from build123d import *

# Parameters (mm, degrees)
F1_DEPTH = 8
F3_DEPTH = 1
F5_DEPTH = 25


with BuildPart() as f1:
    # F0 (on Top) → F1 (new body)
    with BuildSketch(Plane.XY):
        with BuildLine():
            Line((77.8597715207, -29.7489808303), (77.8597715207, 29.7489808303))
            Line((77.8597715207, 29.7489808303), (-77.8597715207, 29.7489808303))
            Line((-77.8597715207, 29.7489808303), (-77.8597715207, -29.7489808303))
            Line((-77.8597715207, -29.7489808303), (-67.8597715207, -29.7489808303))
            Line((-67.8597715207, -29.7489808303), (-67.8597715207, -16.2489808303))
            ThreePointArc((-67.8597715207, -16.2489808303), (-68.9204316925, -13.6883206586), (-66.3597715207, -14.7489808303))
            Line((-66.3597715207, -14.7489808303), (-41.3597715207, -14.7489808303))
            ThreePointArc((-41.3597715207, -14.7489808303), (-38.7991113489, -13.6883206586), (-39.8597715207, -16.2489808303))
            Line((-39.8597715207, -16.2489808303), (-39.8597715207, -29.7489808303))
            Line((-39.8597715207, -29.7489808303), (77.8597715207, -29.7489808303))
        make_face()
        with BuildLine():
            Line((-67.8597715207, -29.7489808303), (-39.8597715207, -29.7489808303))
            Line((-39.8597715207, -29.7489808303), (-39.8597715207, -16.2489808303))
            ThreePointArc((-39.8597715207, -16.2489808303), (-38.7991113489, -13.6883206586), (-41.3597715207, -14.7489808303))
            Line((-41.3597715207, -14.7489808303), (-66.3597715207, -14.7489808303))
            ThreePointArc((-66.3597715207, -14.7489808303), (-68.9204316925, -13.6883206586), (-67.8597715207, -16.2489808303))
            Line((-67.8597715207, -16.2489808303), (-67.8597715207, -29.7489808303))
        make_face()
    extrude(amount=F1_DEPTH)

    # F2 (on face) → F3 (join)
    with BuildSketch(Plane.XY.offset(8)):
        with BuildLine():
            Line((-67.8597715207, -16.2489808303), (-67.8597715207, -29.7489808303))
            Line((-67.8597715207, -29.7489808303), (-39.8597715207, -29.7489808303))
            Line((-39.8597715207, -29.7489808303), (-39.8597715207, -16.2489808303))
            ThreePointArc((-39.8597715207, -16.2489808303), (-38.7991113489, -13.6883206586), (-41.3597715207, -14.7489808303))
            Line((-41.3597715207, -14.7489808303), (-66.3597715207, -14.7489808303))
            ThreePointArc((-66.3597715207, -14.7489808303), (-68.9204316925, -13.6883206586), (-67.8597715207, -16.2489808303))
        make_face()
    extrude(amount=F3_DEPTH)

    # F4 (on face) → F5 (cut)
    with BuildSketch(Plane.XY.offset(9)):
        with BuildLine():
            ThreePointArc((-62.6597715207, -18.936415039), (-62.9597715207, -17.7489808303), (-62.6597715207, -16.5615466216))
            ThreePointArc((-62.6597715207, -16.5615466216), (-67.3597715207, -17.7489808303), (-62.6597715207, -18.936415039))
        make_face()
        with BuildLine():
            ThreePointArc((-62.6597715207, -16.5615466216), (-62.435931592, -17.1366083946), (-62.3597715207, -17.7489808303))
            ThreePointArc((-62.3597715207, -17.7489808303), (-62.435931592, -18.361353266), (-62.6597715207, -18.936415039))
            ThreePointArc((-62.6597715207, -18.936415039), (-60.4597715207, -20.2489808303), (-58.2597715207, -18.936415039))
            ThreePointArc((-58.2597715207, -18.936415039), (-58.5597715207, -17.7489808303), (-58.2597715207, -16.5615466216))
            ThreePointArc((-58.2597715207, -16.5615466216), (-60.4597715207, -15.2489808303), (-62.6597715207, -16.5615466216))
        make_face()
        with BuildLine():
            ThreePointArc((-53.8597715207, -16.5615466216), (-56.0597715207, -15.2489808303), (-58.2597715207, -16.5615466216))
            ThreePointArc((-58.2597715207, -16.5615466216), (-58.035931592, -17.1366083946), (-57.9597715207, -17.7489808303))
            ThreePointArc((-57.9597715207, -17.7489808303), (-58.035931592, -18.361353266), (-58.2597715207, -18.936415039))
            ThreePointArc((-58.2597715207, -18.936415039), (-56.0597715207, -20.2489808303), (-53.8597715207, -18.936415039))
            ThreePointArc((-53.8597715207, -18.936415039), (-54.1597715207, -17.7489808303), (-53.8597715207, -16.5615466216))
        make_face()
        with BuildLine():
            ThreePointArc((-49.4597715207, -16.5615466216), (-51.6597715207, -15.2489808303), (-53.8597715207, -16.5615466216))
            ThreePointArc((-53.8597715207, -16.5615466216), (-53.635931592, -17.1366083946), (-53.5597715207, -17.7489808303))
            ThreePointArc((-53.5597715207, -17.7489808303), (-53.635931592, -18.361353266), (-53.8597715207, -18.936415039))
            ThreePointArc((-53.8597715207, -18.936415039), (-51.6597715207, -20.2489808303), (-49.4597715207, -18.936415039))
            ThreePointArc((-49.4597715207, -18.936415039), (-49.7597715207, -17.7489808303), (-49.4597715207, -16.5615466216))
        make_face()
        with BuildLine():
            ThreePointArc((-45.0597715207, -16.5615466216), (-47.2597715207, -15.2489808303), (-49.4597715207, -16.5615466216))
            ThreePointArc((-49.4597715207, -16.5615466216), (-49.235931592, -17.1366083946), (-49.1597715207, -17.7489808303))
            ThreePointArc((-49.1597715207, -17.7489808303), (-49.235931592, -18.361353266), (-49.4597715207, -18.936415039))
            ThreePointArc((-49.4597715207, -18.936415039), (-47.2597715207, -20.2489808303), (-45.0597715207, -18.936415039))
            ThreePointArc((-45.0597715207, -18.936415039), (-45.3597715207, -17.7489808303), (-45.0597715207, -16.5615466216))
        make_face()
        with BuildLine():
            ThreePointArc((-40.3597715207, -17.7489808303), (-42.247399085, -15.3251409016), (-45.0597715207, -16.5615466216))
            ThreePointArc((-45.0597715207, -16.5615466216), (-44.835931592, -17.1366083946), (-44.7597715207, -17.7489808303))
            ThreePointArc((-44.7597715207, -17.7489808303), (-44.835931592, -18.361353266), (-45.0597715207, -18.936415039))
            ThreePointArc((-45.0597715207, -18.936415039), (-42.247399085, -20.1728207591), (-40.3597715207, -17.7489808303))
        make_face()
        with BuildLine():
            ThreePointArc((-57.9597715207, -17.7489808303), (-58.035931592, -17.1366083946), (-58.2597715207, -16.5615466216))
            ThreePointArc((-58.2597715207, -16.5615466216), (-58.5597715207, -17.7489808303), (-58.2597715207, -18.936415039))
            ThreePointArc((-58.2597715207, -18.936415039), (-58.035931592, -18.361353266), (-57.9597715207, -17.7489808303))
        make_face()
        with BuildLine():
            ThreePointArc((-62.6597715207, -18.936415039), (-62.435931592, -18.361353266), (-62.3597715207, -17.7489808303))
            ThreePointArc((-62.3597715207, -17.7489808303), (-62.435931592, -17.1366083946), (-62.6597715207, -16.5615466216))
            ThreePointArc((-62.6597715207, -16.5615466216), (-62.9597715207, -17.7489808303), (-62.6597715207, -18.936415039))
        make_face()
        with BuildLine():
            ThreePointArc((-53.5597715207, -17.7489808303), (-53.635931592, -17.1366083946), (-53.8597715207, -16.5615466216))
            Line((-53.8597715207, -16.5615466216), (-53.8597715207, -18.936415039))
            ThreePointArc((-53.8597715207, -18.936415039), (-53.635931592, -18.361353266), (-53.5597715207, -17.7489808303))
        make_face()
        with BuildLine():
            ThreePointArc((-49.1597715207, -17.7489808303), (-49.235931592, -17.1366083946), (-49.4597715207, -16.5615466216))
            ThreePointArc((-49.4597715207, -16.5615466216), (-49.7597715207, -17.7489808303), (-49.4597715207, -18.936415039))
            ThreePointArc((-49.4597715207, -18.936415039), (-49.235931592, -18.361353266), (-49.1597715207, -17.7489808303))
        make_face()
        with BuildLine():
            ThreePointArc((-44.7597715207, -17.7489808303), (-44.835931592, -17.1366083946), (-45.0597715207, -16.5615466216))
            ThreePointArc((-45.0597715207, -16.5615466216), (-45.3597715207, -17.7489808303), (-45.0597715207, -18.936415039))
            ThreePointArc((-45.0597715207, -18.936415039), (-44.835931592, -18.361353266), (-44.7597715207, -17.7489808303))
        make_face()
        with BuildLine():
            Line((-53.8597715207, -18.936415039), (-53.8597715207, -16.5615466216))
            ThreePointArc((-53.8597715207, -16.5615466216), (-54.1597715207, -17.7489808303), (-53.8597715207, -18.936415039))
        make_face()
        with BuildLine():
            ThreePointArc((-67.8597715207, -16.2489808303), (-66.7991113489, -15.8096410021), (-66.3597715207, -14.7489808303))
            ThreePointArc((-66.3597715207, -14.7489808303), (-68.9204316925, -13.6883206586), (-67.8597715207, -16.2489808303))
        make_face()
        with BuildLine():
            ThreePointArc((-38.3597715207, -14.7489808303), (-39.8597715207, -13.2489808303), (-41.3597715207, -14.7489808303))
            ThreePointArc((-41.3597715207, -14.7489808303), (-40.9204316925, -15.8096410021), (-39.8597715207, -16.2489808303))
            ThreePointArc((-39.8597715207, -16.2489808303), (-38.7991113489, -15.8096410021), (-38.3597715207, -14.7489808303))
        make_face()
    extrude(amount=-F5_DEPTH, mode=Mode.SUBTRACT)


solid = f1.part
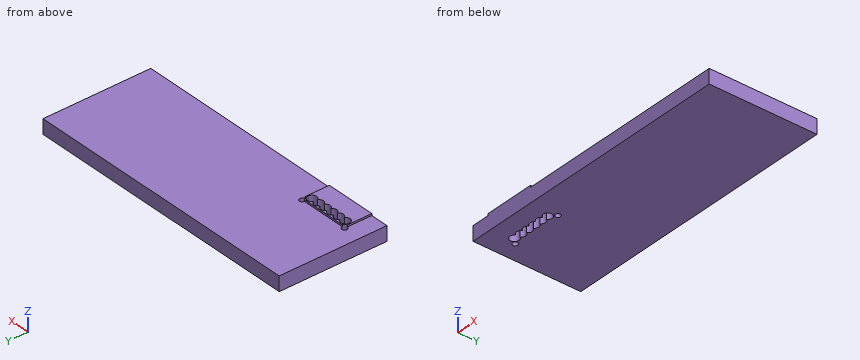
Design review of the part built by this model. Coordinates are the model's own, in mm. Round coordinates to 2 decimals unless told otherwise and drop trailing zeros. Order: outer loops, then holes, each group sorted by start corner. A loop starts at its lowest first (then second) coordinate and runs counter-clockwise, first axis right, second up.
1) For L1, parallel to X at y = -15, z = 5; L2, parallel to Y at x = -64.5, z = 2.5 (3 decimals); L3, parallel to Z at x = 26, y = -13.5, list the stretches that pass through material, from the lowest coordinate up.
The answers:
L1: x = -77.86 to -69.34, -66.38 to -41.34, -38.38 to 77.86
L2: y = -29.749 to -20.223, -15.275 to 29.749
L3: z = 0 to 8
2) Consider section A-A (y = 26). State the section outline as (x, z) points.
The answers:
outline: (-77.86, 0) - (77.86, 0) - (77.86, 8) - (-77.86, 8) - close
3) Consider section B-B (x = -37). State the section outline as (y, z) points, plus the area to 3 significant figures.
The answers:
outline: (-29.75, 0) - (29.75, 0) - (29.75, 8) - (-29.75, 8) - close
area: 476 mm2
4) Clearance check with flat-ended pins moving along their axes: pin 1 Ø0.5 at (y, z) = (-21.5, 8.5) entering from -X; pin 2 Ø0.5 at (y, z) = (-21, 8.5) entering from +X; pin 3 Ø3 at (x, y) = (53.5, 16.5) entering from +Z; pin 4 Ø3 at (x, y) = (-64.86, -17.75) entering from -Z. State where each tip first meets the part, or that it passes through.
The answers:
pin 1: stops at x = -67.86
pin 2: stops at x = -39.86
pin 3: stops at z = 8
pin 4: passes through
